Source: CAD feature listing. Evaluate the final solid. Frame: model axes, mm. A direction names the side the tool comes from. Give positions to 0.01 mm unless a question says otherwise; leave off trailing zeros. Order: outer loops, then holes, each group sorted by start corner. A loop starts at its lowest first (then second) coordinate and runs counter-clockwise, first axis right, second up.
1) Material intervals for line 1 (Z direction, x = 30, y = 26); line 2 (Y direction, x = -15, z = 0.6); line 3 (Y direction, x = 14, z = 0.2), sorted ascending.
2) Access query for faces 4 (the face through (27.89, -27.99, 1.99)), 5 (the face through (-33.289, -33.196, 0.493)), 6 (the face through (25.48, -25.45, 0.49)). Directions: +Z, -Z, +X, -X, +Y, -Y. A direction counts if a zero-diameter tool reaches every point of the face in a straight line with its end or side. Return the directions, or none.
3) Section A-A, the plane y = 0. Give the number of separate pieces and of enclosed holes in the cut face, plus the area to 3 significant figures.
4) Draft query along X for faces 1 (the face through (33.196, -33.289, 0.493)), 2 (the face through (-29, 29, 3)), 3 (the face through (0.1, -26, 0.5)). Return one class per face: released by +X, released by -X, zero draft, split by the parting line, or undercut.
5) First-contact query: P1, Ø2.5, axis at x = 0, y = -29, coming from the +Z side; P2, Ø1.5, axis at y = -16, z = 1, coming from the +X side; P3, Ø3.5, axis at x = 29, y = 0, coming from the +Z side. Flat tips, straight axial feed; report the tip coordinate or a pass-through.
6) Section B-B, the plane z = 2.5. Return loops of the section in (x, y), plus the area to 3 significant figures.
```python
from build123d import *

# Parameters (mm, degrees)
IZIM3_R                          = 1.5
Y_KSEKLIK_EKSTR_ZYON3_DEPTH      = 1
PAH1_SIZE                        = 1
Y_KSEKLIK_EKSTR_ZYON5_DEPTH      = 2
Y_KSEKLIK_EKSTR_ZYON5_DEPTH_BACK = 1
IZIM5_R                          = 1.5
Y_KSEKLIK_EKSTR_ZYON4_DEPTH      = 2
Y_KSEKLIK_EKSTR_ZYON4_DEPTH_BACK = 1
IZIM4_R                          = 1.5


with BuildPart() as part:
    # Çizim3 → Yükseklik-Ekstrüzyon3 (new body)
    with BuildSketch(Plane.XY):
        with BuildLine():
            ThreePointArc((-29, 35), (-33.242640687, 33.242640687), (-35, 29))
            add(Edge.make_bspline(
                [(-35, -29), (-29, 0), (-35, 29)],
                knots=[0, 0, 0, 1, 1, 1], degree=2))
            ThreePointArc((-35, -29), (-33.242640687, -33.242640687), (-29, -35))
            add(Edge.make_bspline(
                [(29, -35), (0, -29), (-29, -35)],
                knots=[0, 0, 0, 1, 1, 1], degree=2))
            ThreePointArc((29, -35), (33.242640687, -33.242640687), (35, -29))
            add(Edge.make_bspline(
                [(35, 29), (29, 0), (35, -29)],
                knots=[0, 0, 0, 1, 1, 1], degree=2))
            ThreePointArc((35, 29), (33.242640687, 33.242640687), (29, 35))
            add(Edge.make_bspline(
                [(-29, 35), (0, 29), (29, 35)],
                knots=[0, 0, 0, 1, 1, 1], degree=2))
        make_face()
        with Locations((0, -29)):
            Circle(IZIM3_R, mode=Mode.SUBTRACT)
        with Locations((-29, 0)):
            Circle(IZIM3_R, mode=Mode.SUBTRACT)
        with Locations((-29, 29)):
            Circle(IZIM3_R, mode=Mode.SUBTRACT)
        with Locations((29, 29)):
            Circle(IZIM3_R, mode=Mode.SUBTRACT)
        with Locations((-29, -29)):
            Circle(IZIM3_R, mode=Mode.SUBTRACT)
        with Locations((29, -29)):
            Circle(IZIM3_R, mode=Mode.SUBTRACT)
        with Locations((0, 29)):
            Circle(IZIM3_R, mode=Mode.SUBTRACT)
        with Locations((29, 0)):
            Circle(IZIM3_R, mode=Mode.SUBTRACT)
        with BuildLine():
            ThreePointArc((-24.479955031, -26.862432812), (-25.464466094, -25.464466094), (-26.862432812, -24.479955031))
            ThreePointArc((-26.862432812, -24.479955031), (-27.257516743, -24.144570316), (-27.431672227, -23.65646778))
            add(Edge.make_bspline(
                [(-27.431672227, -23.65646778), (-28.369214102, -17.081973168), (-28.888327363, -10.491616934), (-28.989012012, -3.885399076)],
                knots=[0, 0, 0, 0, 0.836151593, 0.836151593, 0.836151593, 0.836151593], degree=3))
            ThreePointArc((-28.989012012, -3.885399076), (-28.785191285, -3.264946388), (-28.241846101, -2.902619966))
            ThreePointArc((-28.241846101, -2.902619966), (-26, 0), (-28.241846101, 2.902619966))
            ThreePointArc((-28.241846101, 2.902619966), (-28.785191285, 3.264946388), (-28.989012012, 3.885399076))
            add(Edge.make_bspline(
                [(-27.431672227, 23.65646778), (-28.369214102, 17.081973168), (-28.888327363, 10.491616934), (-28.989012012, 3.885399076)],
                knots=[0, 0, 0, 0, 0.836151593, 0.836151593, 0.836151593, 0.836151593], degree=3))
            ThreePointArc((-27.431672227, 23.65646778), (-27.257516743, 24.144570316), (-26.862432812, 24.479955031))
            ThreePointArc((-26.862432812, 24.479955031), (-25.464466094, 25.464466094), (-24.479955031, 26.862432812))
            ThreePointArc((-24.479955031, 26.862432812), (-24.144570316, 27.257516743), (-23.65646778, 27.431672227))
            add(Edge.make_bspline(
                [(-23.65646778, 27.431672227), (-17.081973168, 28.369214102), (-10.491616934, 28.888327363), (-3.885399076, 28.989012012)],
                knots=[0, 0, 0, 0, 0.836151593, 0.836151593, 0.836151593, 0.836151593], degree=3))
            ThreePointArc((-3.885399076, 28.989012012), (-3.264946388, 28.785191285), (-2.902619966, 28.241846101))
            ThreePointArc((-2.902619966, 28.241846101), (0, 26), (2.902619966, 28.241846101))
            ThreePointArc((2.902619966, 28.241846101), (3.264946388, 28.785191285), (3.885399076, 28.989012012))
            add(Edge.make_bspline(
                [(23.65646778, 27.431672227), (17.081973168, 28.369214102), (10.491616934, 28.888327363), (3.885399076, 28.989012012)],
                knots=[0, 0, 0, 0, 0.836151593, 0.836151593, 0.836151593, 0.836151593], degree=3))
            ThreePointArc((23.65646778, 27.431672227), (24.144570316, 27.257516743), (24.479955031, 26.862432812))
            ThreePointArc((24.479955031, 26.862432812), (25.464466094, 25.464466094), (26.862432812, 24.479955031))
            ThreePointArc((26.862432812, 24.479955031), (27.257516743, 24.144570316), (27.431672227, 23.65646778))
            add(Edge.make_bspline(
                [(27.431672227, 23.65646778), (28.369214102, 17.081973168), (28.888327363, 10.491616934), (28.989012012, 3.885399076)],
                knots=[0, 0, 0, 0, 0.836151593, 0.836151593, 0.836151593, 0.836151593], degree=3))
            ThreePointArc((28.989012012, 3.885399076), (28.785191285, 3.264946389), (28.241846101, 2.902619966))
            ThreePointArc((28.241846101, 2.902619966), (26, 0), (28.241846101, -2.902619966))
            ThreePointArc((28.241846101, -2.902619966), (28.785191285, -3.264946388), (28.989012012, -3.885399076))
            add(Edge.make_bspline(
                [(27.431672227, -23.65646778), (28.369214102, -17.081973168), (28.888327363, -10.491616934), (28.989012012, -3.885399076)],
                knots=[0, 0, 0, 0, 0.836151593, 0.836151593, 0.836151593, 0.836151593], degree=3))
            ThreePointArc((27.431672227, -23.65646778), (27.257516743, -24.144570316), (26.862432812, -24.479955031))
            ThreePointArc((26.862432812, -24.479955031), (25.464466094, -25.464466094), (24.479955031, -26.862432812))
            ThreePointArc((24.479955031, -26.862432812), (24.144570316, -27.257516743), (23.65646778, -27.431672227))
            add(Edge.make_bspline(
                [(23.65646778, -27.431672227), (17.081973168, -28.369214102), (10.491616934, -28.888327363), (3.885399076, -28.989012012)],
                knots=[0, 0, 0, 0, 0.836151593, 0.836151593, 0.836151593, 0.836151593], degree=3))
            ThreePointArc((3.885399076, -28.989012012), (3.264946388, -28.785191285), (2.902619966, -28.241846101))
            ThreePointArc((2.902619966, -28.241846101), (0, -26), (-2.902619966, -28.241846101))
            ThreePointArc((-2.902619966, -28.241846101), (-3.264946388, -28.785191285), (-3.885399076, -28.989012012))
            add(Edge.make_bspline(
                [(-23.65646778, -27.431672227), (-17.081973168, -28.369214102), (-10.491616934, -28.888327363), (-3.885399076, -28.989012012)],
                knots=[0, 0, 0, 0, 0.836151593, 0.836151593, 0.836151593, 0.836151593], degree=3))
            ThreePointArc((-23.65646778, -27.431672227), (-24.144570316, -27.257516743), (-24.479955031, -26.862432812))
        make_face(mode=Mode.SUBTRACT)
    extrude(amount=Y_KSEKLIK_EKSTR_ZYON3_DEPTH)

    # Pah1
    pah1_edges = [part.edges().sort_by_distance(p)[0] for p in [
        (-1.5, 29, 1),
        (27.5, 0, 1),
        (-1.5, -29, 1),
        (-30.5, 0, 1),
    ]]
    chamfer(pah1_edges, length=PAH1_SIZE - 0.0001)  # a hair under: the kernel refuses the full size

    # Çizim5 → Yükseklik-Ekstrüzyon5 (add, two sides: drawn at the far end of the back side and taken through both)
    with BuildSketch(Plane.XY.offset(1).offset(-Y_KSEKLIK_EKSTR_ZYON5_DEPTH_BACK)):
        with Locations((-29, 29)):
            Circle(IZIM5_R)
        with Locations((29, 29)):
            Circle(IZIM5_R)
        with Locations((29, -29)):
            Circle(IZIM5_R)
        with Locations((-29, -29)):
            Circle(IZIM5_R)
    extrude(amount=Y_KSEKLIK_EKSTR_ZYON5_DEPTH + Y_KSEKLIK_EKSTR_ZYON5_DEPTH_BACK)

    # Çizim4 → Yükseklik-Ekstrüzyon4 (add, two sides: drawn at the far end of the back side and taken through both)
    with BuildSketch(Plane.XY.offset(1).offset(-Y_KSEKLIK_EKSTR_ZYON4_DEPTH_BACK)):
        with Locations((-29, 29)):
            Circle(IZIM4_R)
        with Locations((29, 29)):
            Circle(IZIM4_R)
        with Locations((29, -29)):
            Circle(IZIM4_R)
        with Locations((-29, -29)):
            Circle(IZIM4_R)
    extrude(amount=Y_KSEKLIK_EKSTR_ZYON4_DEPTH + Y_KSEKLIK_EKSTR_ZYON4_DEPTH_BACK)


solid = part.part
```
From the geometry:
1. line 1: z = 0 to 1
1. line 2: y = -32.8 to -28.42, 28.42 to 32.8
1. line 3: y = -32.7 to -28.51, 28.51 to 32.7
2. face 4: +Z
2. face 5: +Z, -Z, -X, -Y
2. face 6: +Z, -Z
3. separate pieces: 4
3. enclosed holes: 0
3. area: 4.00 mm2
4. face 1: released by +X
4. face 2: zero draft
4. face 3: undercut
5. P1: passes through
5. P2: stops at x = 33
5. P3: stops at z = 0.25
6. outline: circle Ø3 at (-29, -29); circle Ø3 at (-29, 29); circle Ø3 at (29, -29); circle Ø3 at (29, 29)
6. area: 28.3 mm2
